Can you work these out from the model? Positions are in its coordinate system, mm. A direction names the side the tool comes from. Round coordinates to 2 decimals unless told otherwise and drop trailing zeros. Order: outer loops, then holes, each group sorted by start corner. A loop starts at its lowest first (then second) coordinate and runs counter-clockwise, first axis right, second up. Notation, with made-up numbers: M -2.5,-1 L 42.5,-1 A21 cw 42.5,30 Z; hole C 2.25,49 d3. An arc over 180 degrees is marked long. One line per question, with ' | ' between items.
```python
from build123d import *

# Parameters (mm, degrees)
F0_W     = 6.35
F0_H     = 25.4
F0_R     = 17.5576306553
F1_DEPTH = 6.35
F2_R     = 1.27
F3_W     = 6.35
F3_H     = 25.4
F4_DEPTH = 5.08
F5_R     = 1.27


# Not quite as in the source:
# - a feature names something its author has since deleted; it is built from what else it names


with BuildPart() as f1:
    # F0 (on Top) → F1 (new body)
    with BuildSketch(Plane.XY):
        with BuildLine():
            ThreePointArc((101.6, 13.97), (99.7401280605, 18.4601280605), (95.25, 20.32))
            Line((95.25, 20.32), (-95.25, 20.32))
            ThreePointArc((-95.25, 20.32), (-99.7401280605, 18.4601280605), (-101.6, 13.97))
            Line((-101.6, 13.97), (-101.6, -13.97))
            ThreePointArc((-101.6, -13.97), (-99.7401280605, -18.4601280605), (-95.25, -20.32))
            Line((-95.25, -20.32), (95.25, -20.32))
            ThreePointArc((95.25, -20.32), (99.7401280605, -18.4601280605), (101.6, -13.97))
            Line((101.6, -13.97), (101.6, 13.97))
        make_face()
        with Locations((-90.6151607633, 0)):
            Rectangle(F0_W, F0_H, mode=Mode.SUBTRACT)
        with Locations((-77.9151607633, 0)):
            Rectangle(F0_W, F0_H, mode=Mode.SUBTRACT)
        with Locations((-65.2151607633, 0)):
            Rectangle(F0_W, F0_H, mode=Mode.SUBTRACT)
        with Locations((-52.5151607633, 0)):
            Rectangle(F0_W, F0_H, mode=Mode.SUBTRACT)
        with Locations((-39.8151607633, 0)):
            Rectangle(F0_W, F0_H, mode=Mode.SUBTRACT)
        with Locations((4.1378471069, 0)):
            Circle(F0_R, mode=Mode.SUBTRACT)
        with Locations((4.1378471069, 0)):
            Circle(F0_R)
    extrude(amount=F1_DEPTH)

    # F2
    f2_edges = [f1.edges().sort_by_distance(p)[0] for p in [
        (0, -20.32, 0),
        (0, -20.32, 6.35),
    ]]
    fillet(f2_edges, radius=F2_R)

    # F3 (on face) → F4 (join)
    with BuildSketch(Plane.XY.offset(6.35)):
        with Locations((78.503764081, 0)):
            Rectangle(F3_W, F3_H)
        with Locations((91.203764081, 0)):
            Rectangle(F3_W, F3_H)
    extrude(amount=F4_DEPTH)

    # F5
    f5_edges = [f1.edges().sort_by_distance(p)[0] for p in [
        (81.678764, 0, 11.43),
        (78.503764, -12.7, 11.43),
        (75.328764, 0, 11.43),
        (78.503764, 12.7, 11.43),
        (88.028764, 0, 11.43),
        (94.378764, 0, 11.43),
        (91.203764, -12.7, 11.43),
        (91.203764, 12.7, 11.43),
        (94.378764, -12.7, 8.89),
        (88.028764, -12.7, 8.89),
        (81.678764, -12.7, 8.89),
        (75.328764, -12.7, 8.89),
        (81.678764, 12.7, 8.89),
        (94.378764, 12.7, 8.89),
        (88.028764, 12.7, 8.89),
        (75.328764, 12.7, 8.89),
    ]]
    fillet(f5_edges, radius=F5_R)


solid = f1.part
```
(1) If we section it at A-A on x = -79: Please give me the cut outline in (y, z).
Final values:
outline: M -20.32,1.27 A1.27 ccw -19.05,0 L -12.7,0 L -12.7,6.35 L -19.05,6.35 A1.27 ccw -20.32,5.08 Z; M 12.7,0 L 19.05,0 A1.27 ccw 20.32,1.27 L 20.32,5.08 A1.27 ccw 19.05,6.35 L 12.7,6.35 Z
(2) Thinking about a two-plate mould opening in Y: for faces 1 (the flat face through (-68.39, 0, 3)), 2 (the cylindrical face through (-99.7, 18.5, 3.1)), 3 (the cylindrical face through (99.7, -18.5, 3.1)), which applies, released by +Y, released by -Y, zero draft, split by the parting line, or undercut?
Final values:
face 1: undercut | face 2: released by +Y | face 3: released by -Y
(3) If we section it at B-B on x = 25.5: Please give me the cut outline in (y, z).
Final values:
outline: M -20.32,1.27 A1.27 ccw -19.05,0 L 19.05,0 A1.27 ccw 20.32,1.27 L 20.32,5.08 A1.27 ccw 19.05,6.35 L -19.05,6.35 A1.27 ccw -20.32,5.08 Z
(4) If we section it at C-C on y = 6.5: State how many separate pieces and enclosed holes the cut face has, plus the area to 3 significant figures.
Final values:
separate pieces: 6 | enclosed holes: 0 | area: 1,150 mm^2
(5) Will these pins go through, and if not, where does the flat tip stop? pin 1 Ø1.9 at (x, z) = (77.5, 7.5) entering from +Y; pin 2 Ø1 at (y, z) = (10, 10) entering from -X; pin 3 Ø1.9 at (x, z) = (78.5, 8.5) entering from -Y.
Final values:
pin 1: y = 12.7 | pin 2: x = 75.33 | pin 3: y = -12.7
(6) On a 3-axis mill with a long thin cutter (end or side, diameter ignored), from which of +Z, -Z, +X, -X, +Y, -Y can I reach the whole of each face in a straight line? I mean faces 4 (the flat face through (78, -12.7, 8)), 5 (the flat face through (-49.34, 0, 3)), 6 (the flat face through (81.679, 0, 8)). Say none if no direction works.
Final values:
face 4: +Z, +X, -X, -Y | face 5: +Z, -Z | face 6: +Z, +Y, -Y
(7) Please list where these lines run through material, in increasing order: probe 1 along X at (y, z) = (-5.5, 2.75); probe 2 along Y at (x, z) = (-64.5, 4.5); probe 3 along Z at (x, y) = (68, 13). Write a range as [from, to].
Final values:
probe 1: [-101.6, -93.79], [-87.44, -81.09], [-74.74, -68.39], [-62.04, -55.69], [-49.34, -42.99], [-36.64, 101.6] | probe 2: [-20.32, -12.7], [12.7, 20.32] | probe 3: [0, 6.35]
